Geometry: final body of the model. Coordinates: model frame, mm. A direction names the side the tool comes from. Give positions to 0.01 mm unless a question says otherwise; leave off trailing zeros. Write each loop counter-clockwise with the first axis right and the second up, starting at its lowest first coordinate (ties: lowest second). Pieces come first, ordered by that corner, then holes. Notation, with made-up numbers: (8, 10.5) -> (14, 10.5) arc R36 cw to (14, 45.5) -> close; hole circle Ø8 at (-40, 21.25). An arc over 180 degrees is marked (long way). Answer as a JSON object with one key per item and string values. Group by question number.
(1) Material intervals for probe 1 along Y at (x, z) = (10, 1); probe 2 along X at (y, z) = (2.25, 6.5); probe 3 along Z at (x, y) = (-12, -0.25), sorted ascending.
(2) Section query C-C on z = 1.5. Output: boundary loops of the cut face in (x, y), plus the area to 3 significant figures.
(3) Section query D-D on x = -9. Output: boundary loops of the cut face in (y, z).
(4) Section query A-A on y = 1.5. Output: boundary loops of the cut face in (x, z).
(5) Draft query along Z for faces 4 (the face through (9, 2, 1)), 5 (the face through (8.263, 1.479, 5.676)), 6 (the face through (-9.737, 1.479, 5.676)), 7 (the face through (-13, 1, 1)). Return one class per face: +Z half, -Z half, draft (parallel to the pull), parting line (faces both ways), or undercut.
(6) Section query B-B on z = 5. Output: boundary loops of the cut face in (x, y).
(7) Contact query for flat-ended pins moving along their axis: pin 1 Ø2.5 at (y, z) = (1.5, 5.5) entering from +X; pin 2 Ø1.5 at (y, z) = (1.5, 2.5) entering from -X; pin 3 Ø4 at (y, z) = (0, 3) entering from +X; pin 4 Ø0.8 at (x, z) = (-15, 1) entering from +Y. Output: stop coordinate, or through.
(8) Set-up query: faces 1 (the face through (-6, 1, 4)), 2 (the face through (8.5, -3.93, 0.99)), 3 (the face through (15, 0, 1)). Return all of +Z, -Z, +X, -X, +Y, -Y with unobstructed straight access to the full face (end or side cutting, diameter ignored); none if empty.
from build123d import *

# Parameters (mm, degrees)
F0_R     = 1.5
F1_DEPTH = 2
F2_W     = 6
F2_H     = 8
F2_R     = 1
F3_DEPTH = 3
F4_SIZE  = 2
F5_SIZE  = 2


with BuildPart() as f1:
    # F0 (on Top) → F1 (new body)
    with BuildSketch(Plane.XY):
        with BuildLine():
            Line((-6.5, 0), (-15.5, 0))
            Line((-15.5, 0), (-15.5, -9.5))
            Line((-15.5, -9.5), (15.5, -9.5))
            Line((15.5, -9.5), (15.5, 0))
            Line((15.5, 0), (6.5, 0))
            ThreePointArc((6.5, 0), (0, -3.3363104735), (-6.5, 0))
        make_face()
        with Locations((-10, -4)):
            Circle(F0_R, mode=Mode.SUBTRACT)
        with Locations((10, -4)):
            Circle(F0_R, mode=Mode.SUBTRACT)
    extrude(amount=F1_DEPTH)

    # F2 (on Front) → F3 (join)
    with BuildSketch(Plane.XZ):
        with Locations((-9, 4)):
            Rectangle(F2_W, F2_H)
        with Locations((-9, 5)):
            Circle(F2_R, mode=Mode.SUBTRACT)
        with Locations((9, 4)):
            Rectangle(F2_W, F2_H)
        with Locations((9, 5)):
            Circle(F2_R, mode=Mode.SUBTRACT)
    extrude(amount=-F3_DEPTH)

    # F4
    f4_edges = [f1.edges().sort_by_distance(p)[0] for p in [
        (9, 3, 0),
        (-9, 3, 0),
    ]]
    chamfer(f4_edges, length=F4_SIZE)

    # F5
    f5_edges = [f1.edges().sort_by_distance(p)[0] for p in [
        (-12, 0, 1),
        (12, 0, 1),
    ]]
    chamfer(f5_edges, length=F5_SIZE)


solid = f1.part
Answer list:
{
 "1": {"probe 1": "-9.5 to -5.5, -2.5 to 2", "probe 2": "-12 to -6, 6 to 12", "probe 3": "0 to 2"},
 "2": {"outline": "(-15.5, -9.5) -> (15.5, -9.5) -> (15.5, 0) -> (14, 0) -> (12, 2) -> (12, 2.5) -> (6, 2.5) -> (6, 0) -> (6.5, 0) arc R8 cw to (-6.5, 0) -> (-6, 0) -> (-6, 2.5) -> (-12, 2.5) -> (-12, 2) -> (-14, 0) -> (-15.5, 0) -> close; hole circle Ø3 at (-10, -4); hole circle Ø3 at (10, -4)", "area": "284 mm2"},
 "3": {"outline": "(-9.5, 0) -> (-5.12, 0) -> (-5.12, 2) -> (-9.5, 2) -> close; (-2.88, 0) -> (1, 0) -> (3, 2) -> (3, 4) -> (0, 4) -> (0, 2) -> (-2.88, 2) -> close; (0, 6) -> (3, 6) -> (3, 8) -> (0, 8) -> close"},
 "4": {"outline": "(-12.5, 0.5) -> (-6, 0.5) -> (-6, 8) -> (-12, 8) -> (-12, 2) -> (-12.5, 2) -> close; (6, 0.5) -> (12.5, 0.5) -> (12.5, 2) -> (12, 2) -> (12, 8) -> (6, 8) -> close; hole circle Ø2 at (-9, 5); hole circle Ø2 at (9, 5)"},
 "5": {"face 4": "-Z half", "face 5": "undercut", "face 6": "undercut", "face 7": "draft"},
 "6": {"outline": "(-12, 0) -> (-10, 0) -> (-10, 3) -> (-12, 3) -> close; (-8, 0) -> (-6, 0) -> (-6, 3) -> (-8, 3) -> close; (6, 0) -> (8, 0) -> (8, 3) -> (6, 3) -> close; (10, 0) -> (12, 0) -> (12, 3) -> (10, 3) -> close"},
 "7": {"pin 1": "x = 12", "pin 2": "x = -13.06", "pin 3": "x = 15.5", "pin 4": "y = 0"},
 "8": {"face 1": "+Z, -Z, +Y", "face 2": "+Z, -Z", "face 3": "+Z, -Z, +X, +Y"}
}
